Can you work these out from the model? Positions are in its coordinate system, mm. A direction names the side the tool comes from. Round coordinates to 2 decimals unless told otherwise and drop trailing zeros. Write each loop counter-clockwise with the first axis right and the second up, starting at its lowest first coordinate (ties: lowest second). Pieces come first, ordered by that corner, then holes. Notation, with made-up numbers: (46, 52.25) -> (98, 52.25) arc R17 ccw to (98, 74.25) -> close; hole circle Ø11 at (32, -23.75). An arc over 180 degrees is marked (long way). Use CSV: the item, a comma, the result in double quotes.
```python
from build123d import *

# Parameters (mm, degrees)
SKETCH1_R           = 2
BOSS_EXTRUDE1_DEPTH = 2.5
FILLET1_R           = 5
BOSS_EXTRUDE2_DEPTH = 1
BOSS_EXTRUDE3_DEPTH = 16
FILLET2_R           = 2
CUT_EXTRUDE1_DEPTH  = 18
FILLET3_R           = 1
BOSS_EXTRUDE4_START = 8
BOSS_EXTRUDE4_DEPTH = 10


with BuildPart() as part:
    # Sketch1 → Boss-Extrude1 (new body)
    with BuildSketch(Plane(origin=(0, 0, 0), x_dir=(1, 0, 0), z_dir=(0, 1, 0))):
        Polygon((25, 0), (14, -29), (0, -29), (0, 29), (14, 29), align=None)
        with Locations((19.1, 0)):
            Circle(SKETCH1_R, mode=Mode.SUBTRACT)
    extrude(amount=-BOSS_EXTRUDE1_DEPTH)

    # Fillet1
    fillet1_edges = [part.edges().sort_by_distance(p)[0] for p in [
        (14, -1.25, -29),
        (25, -1.25, 0),
        (14, -1.25, 29),
    ]]
    fillet(fillet1_edges, radius=FILLET1_R)

    # Sketch2 → Boss-Extrude2 (add)
    with BuildSketch(Plane(origin=(0, 0, 0), x_dir=(1, 0, 0), z_dir=(0, 1, 0))):
        with BuildLine():
            Line((0, 27), (11, 27))
            ThreePointArc((11, 27), (13.121320344, 26.121320344), (14, 24))
            Line((14, 24), (14, -24))
            ThreePointArc((14, -24), (13.121320344, -26.121320344), (11, -27))
            Line((11, -27), (0, -27))
            Line((0, -27), (0, 27))
        make_face()
    extrude(amount=BOSS_EXTRUDE2_DEPTH)

    # Sketch3 → Boss-Extrude3 (add)
    with BuildSketch(Plane.XZ.offset(2.5)):
        Polygon((0, 23.5), (13.5, 23.5), (13.5, -17.5), (7.5, -23.5), (0, -23.5), align=None)
    extrude(amount=BOSS_EXTRUDE3_DEPTH)

    # Fillet2
    fillet2_edges = [part.edges().sort_by_distance(p)[0] for p in [
        (13.5, -10.5, -17.5),
        (7.5, -10.5, -23.5),
        (13.5, -10.5, 23.5),
    ]]
    fillet(fillet2_edges, radius=FILLET2_R)

    # Sketch5 → Cut-Extrude1 (cut)
    with BuildSketch(Plane(origin=(0, 1, 0), x_dir=(1, 0, 0), z_dir=(0, 1, 0))):
        Polygon((0, 22.2), (7, 22.2), (12, 17.2), (12, 5.3), (0, 5.3), align=None)
    extrude(amount=-CUT_EXTRUDE1_DEPTH, mode=Mode.SUBTRACT)

    # Fillet3
    fillet3_edges = [part.edges().sort_by_distance(p)[0] for p in [
        (7, -8, -22.2),
        (12, -8, -17.2),
        (12, -8, -5.3),
    ]]
    fillet(fillet3_edges, radius=FILLET3_R)

    # Mirror1: part across plane


with BuildPart() as part_1:
    add(part.part)
    add(part.part.mirror(Plane(origin=(0, -2.5, -29), x_dir=(0, 0, 1), z_dir=(-1, 0, 0))))

    # Sketch6 → Boss-Extrude4 (add)
    with BuildSketch(Plane.XY.offset(BOSS_EXTRUDE4_START)):
        with BuildLine():
            Line((-9, 1), (-5.383132121, 5.683158511))
            ThreePointArc((-5.383132121, 5.683158511), (-4.605403481, 6.071821883), (-3.817307634, 5.704635295))
            ThreePointArc((-3.817307634, 5.704635295), (2.199237296, 2.28405626), (9, 1))
            Line((9, 1), (-9, 1))
        make_face()
    extrude(amount=BOSS_EXTRUDE4_DEPTH)


solid = part_1.part
```
Q1. On a 3-axis mill with a long thin cutter (end or side, diameter ignored), from which of +Z, -Z, +X, -X, +Y, -Y can I reach the whole of each face in a straight line? I mean faces 1 (the face through (12, -8, -12)), 2 (the face through (-12.93, -10.61, 22.9)), 3 (the face through (-4, 2, 8)), 4 (the face through (-11, -10, -20)). Say none if no direction works.
Resolved:
face 1,"+Y"
face 2,"+Z, -X, -Y"
face 3,"-Z, +X, -X, +Y"
face 4,"-Z, -X, -Y"
Q2. Suppose I cut it at A-A (z = 0). Write out the boundary of the cut face in (x, y).
Resolved:
outline,"(-24.65, -2.5) -> (-21.1, -2.5) -> (-21.1, 0) -> (-24.65, 0) -> close; (-17.1, -2.5) -> (-13.5, -2.5) -> (-13.5, -18.5) -> (13.5, -18.5) -> (13.5, -2.5) -> (17.1, -2.5) -> (17.1, 0) -> (14, 0) -> (14, 1) -> (-14, 1) -> (-14, 0) -> (-17.1, 0) -> close; (21.1, -2.5) -> (24.65, -2.5) -> (24.65, 0) -> (21.1, 0) -> close"
Q3. Suppose I cut it at D-D (z = 16.5). Write out the boundary of the cut face in (x, y).
Resolved:
outline,"(-18.74, -2.5) -> (-13.5, -2.5) -> (-13.5, -18.5) -> (13.5, -18.5) -> (13.5, -2.5) -> (18.74, -2.5) -> (18.74, 0) -> (14, 0) -> (14, 1) -> (9, 1) arc R21.05 cw to (-3.82, 5.7) arc R1 ccw to (-5.38, 5.68) -> (-9, 1) -> (-14, 1) -> (-14, 0) -> (-18.74, 0) -> close"
Q4. Suppose I cut it at B-B (y = -5.5). Write out the boundary of the cut face in (x, z), and give its area (3 significant figures).
Resolved:
outline,"(-13.5, -16.67) arc R2 ccw to (-12.91, -18.09) -> (-8.09, -22.91) arc R2 ccw to (-6.67, -23.5) -> (6.67, -23.5) arc R2 ccw to (8.09, -22.91) -> (12.91, -18.09) arc R2 ccw to (13.5, -16.67) -> (13.5, 21.5) arc R2 ccw to (11.5, 23.5) -> (-11.5, 23.5) arc R2 ccw to (-13.5, 21.5) -> close; hole (-12, -16.79) arc R1 ccw to (-11.71, -17.49) -> (-7.29, -21.91) arc R1 ccw to (-6.59, -22.2) -> (6.59, -22.2) arc R1 ccw to (7.29, -21.91) -> (11.71, -17.49) arc R1 ccw to (12, -16.79) -> (12, -6.3) arc R1 ccw to (11, -5.3) -> (-11, -5.3) arc R1 ccw to (-12, -6.3) -> close"
area,"851 mm^2"
Q5. If we mould it in two halves opening along Z, with no side actions, what happens to faces 5 (the face through (2.108, 2.318, 12.93)), 6 (the face through (0, -17, -14)), 7 (the face through (-13.424, -1.268, 28.091))? For each: released by +Z, released by -Z, zero draft, split by the parting line, or undercut.
Resolved:
face 5,"zero draft"
face 6,"undercut"
face 7,"released by +Z"
Q6. Will these pins go through, and if not, where does the flat tip stop? P1, Ø6, axis at x = 16.5, y = -4, coming from the -Z side; P2, Ø5, axis at x = 9, y = -6, coming from the -Z side; P3, Ø0.5, axis at x = 1.5, y = 0.5, coming from the -Z side; P4, Ø8, axis at x = -6.5, z = 19, coming from the +Y side.
Resolved:
P1,"stops at z = -27.71"
P2,"stops at z = -23.5"
P3,"stops at z = -27"
P4,"stops at y = 6.07"
Q7. Please list where these lines run through material, in increasing order: probe 1 along X at (y, z) = (-0.75, 0); probe 2 along X at (y, z) = (-16.25, -9); probe 3 along Z at (x, y) = (6, -7.25).
Resolved:
probe 1,"x = -24.65 to -21.1, -17.1 to 17.1, 21.1 to 24.65"
probe 2,"x = -13.5 to -12, 12 to 13.5"
probe 3,"z = -23.5 to -22.2, -5.3 to 23.5"
Q8. Suppose I cut it at C-C (x = 19.1). Write out the boundary of the cut face in (y, z).
Resolved:
outline,"(-2.5, -15.55) -> (0, -15.55) -> (0, -2) -> (-2.5, -2) -> close; (-2.5, 2) -> (0, 2) -> (0, 15.55) -> (-2.5, 15.55) -> close"
